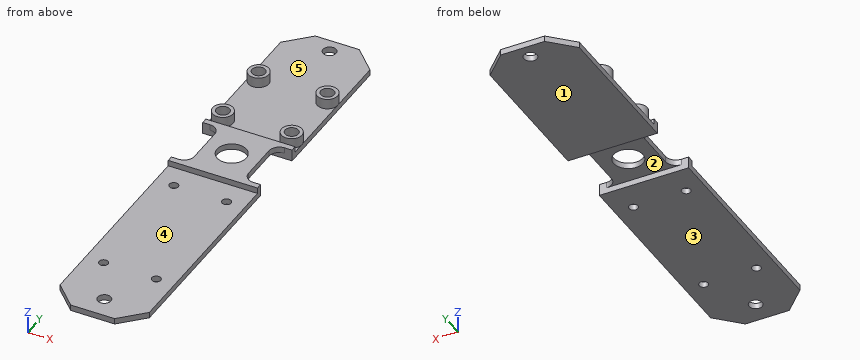
from build123d import *

# Parameters (mm, degrees)
SKETCH_1_W                   = 157.5
SKETCH_1_H                   = 30.5
EXTRUDE_1_DEPTH              = 2
HOLE_WIZARD_4_5_3_05_1_D     = 3.05
HOLE_WIZARD_4_5_3_05_1_DEPTH = 2.5
SKETCH_4_R                   = 3.5
EXTRUDE_2_DEPTH              = 3.5
SKETCH_5_R                   = 2.275
CUT_EXTRUDE_1_DEPTH          = 3.5
SKETCH_6_W                   = 30.5
SKETCH_6_H                   = 20.2
CUT_EXTRUDE_3_DEPTH          = 2.1
SKETCH_9_W                   = 30.5
SKETCH_9_H                   = 24.2
EXTRUDE_6_DEPTH              = 2
SKETCH_12_R                  = 5
CUT_EXTRUDE_4_DEPTH          = 6.5
HOLE_WIZARD_M4_1_D           = 4.5
SKETCH_13_W                  = 6
SKETCH_13_H                  = 20.2
CUT_EXTRUDE_5_DEPTH          = 4.5
FILLET_8_R                   = 3.5
CHAMFER_1_SIZE               = 7.75


with BuildPart() as part:
    # ｽｹｯﾁ1 → ﾎﾞｽ - 押し出し1 (new body)
    with BuildSketch(Plane(origin=(0, 0, 0), x_dir=(0, 1, 0), z_dir=(0, 0, 1))):
        with Locations((78.75, 15.25)):
            Rectangle(SKETCH_1_W, SKETCH_1_H)
    extrude(amount=EXTRUDE_1_DEPTH)

    # Ø4.5 (3.05) 直径の穴1
    with Locations(Plane.XY.offset(2)):
        with Locations((-24.25, 24), (-6.25, 69.2), (-24.25, 69.2), (-6.25, 24)):
            Hole(HOLE_WIZARD_4_5_3_05_1_D / 2, depth=HOLE_WIZARD_4_5_3_05_1_DEPTH)

    # ｽｹｯﾁ4 → ﾎﾞｽ - 押し出し2 (add)
    with BuildSketch(Plane.XY.offset(2)):
        with Locations((-27, 129)):
            Circle(SKETCH_4_R)
        with Locations((-3.5, 129)):
            Circle(SKETCH_4_R)
        with Locations((-3.5, 106)):
            Circle(SKETCH_4_R)
        with Locations((-27, 106)):
            Circle(SKETCH_4_R)
    extrude(amount=EXTRUDE_2_DEPTH)

    # ｽｹｯﾁ5 → ｶｯﾄ - 押し出し1 (cut)
    with BuildSketch(Plane.XY.offset(5.5)):
        with Locations((-27, 129)):
            Circle(SKETCH_5_R)
        with Locations((-3.5, 129)):
            Circle(SKETCH_5_R)
        with Locations((-3.5, 106)):
            Circle(SKETCH_5_R)
        with Locations((-27, 106)):
            Circle(SKETCH_5_R)
    extrude(amount=-CUT_EXTRUDE_1_DEPTH, mode=Mode.SUBTRACT)

    # ｽｹｯﾁ6 → ｶｯﾄ - 押し出し3 (cut)
    with BuildSketch(Plane(origin=(0, 0, 0), x_dir=(1, 0, 0), z_dir=(0, 0, -1))):
        with Locations((-15.25, -89.5)):
            Rectangle(SKETCH_6_W, SKETCH_6_H)
    extrude(amount=-CUT_EXTRUDE_3_DEPTH, mode=Mode.SUBTRACT)

    # ｽｹｯﾁ9 → ﾎﾞｽ - 押し出し6 (add)
    with BuildSketch(Plane.XY.offset(2)):
        with Locations((-15.25, 89.5)):
            Rectangle(SKETCH_9_W, SKETCH_9_H)
    extrude(amount=EXTRUDE_6_DEPTH)

    # ｽｹｯﾁ12 → ｶｯﾄ - 押し出し4 (cut, through all)
    with BuildSketch(Plane.XY.offset(5.5)):
        with Locations((-15.25, 89.5)):
            Circle(SKETCH_12_R)
    extrude(amount=-CUT_EXTRUDE_4_DEPTH, mode=Mode.SUBTRACT)

    # M4 すきま穴1 (through all)
    with Locations(Plane.XY.offset(2)):
        with Locations((-15.25, 152.5), (-15.25, 7.5)):
            Hole(HOLE_WIZARD_M4_1_D / 2)

    # ｽｹｯﾁ13 → ｶｯﾄ - 押し出し5 (cut, through all)
    with BuildSketch(Plane(origin=(0, 0, 2), x_dir=(1, 0, 0), z_dir=(0, 0, -1))):
        with Locations((-3, -89.5)):
            Rectangle(SKETCH_13_W, SKETCH_13_H)
        with Locations((-27.5, -89.5)):
            Rectangle(SKETCH_13_W, SKETCH_13_H)
    extrude(amount=-CUT_EXTRUDE_5_DEPTH, mode=Mode.SUBTRACT)

    # ﾌｨﾚｯﾄ8
    fillet_8_edges = [part.edges().sort_by_distance(p)[0] for p in [
        (-6, 99.6, 3),
        (-6, 79.4, 3),
        (-24.5, 79.4, 3),
        (-24.5, 99.6, 3),
    ]]
    fillet(fillet_8_edges, radius=FILLET_8_R)

    # 面取り1
    chamfer_1_edges = [part.edges().sort_by_distance(p)[0] for p in [
        (0, 157.5, 1),
        (-30.5, 157.5, 1),
        (-30.5, 0, 1),
        (0, 0, 1),
    ]]
    chamfer(chamfer_1_edges, length=CHAMFER_1_SIZE)


solid = part.part
The listing builds one solid part. Answer for the finished solid, in the listing's coordinates (mm). Face numbers are marked on the shaded views. A direction names the side the tool comes from. Give positions to 0.01 mm unless a question says otherwise; leave off trailing zeros. Write each loop counter-clockwise with the first axis right and the second up, starting at its lowest first coordinate (ties: lowest second). Pieces come first, ordered by that corner, then holes. Notation, with made-up numbers: (-39.5, -4) -> (-18.5, -4) arc R20 cw to (-18.5, 32) -> close; hole circle Ø3 at (66, 23.25). An arc over 180 degrees is marked (long way). One line per question, with ' | ' between items. Start each with the question number.
1. Section A-A (y = 89.5) is taken. Determine the outline of the cut face in (x, z), plus the area to 3 significant figures.
2. Section D-D (y = 142.5) is taken. Determine the outline of the cut face in (x, z), plus the area to 3 significant figures.
3. For a pull along Y with two mould halves and no side action, classify the marked faces 1 and 2 as pulls with the +Y half, pulls with the -Y half, needs draft (parallel to the pull), parting line crosses it, or undercut.
4. Find the intervals of material crossed by probe 1 along Y at (x, z) = (-15.25, 0.7); probe 2 along Y at (x, z) = (-5, 1.6); probe 3 along Y at (x, z) = (-22.5, 1.6), in increasing order.
5. For the marked faces 3, 4 and 5, determine the directions among +Z, -Z, +X, -X, +Y, -Y from which every point of the face is accessible in a straight line to the end or side of a thin tool.
6. Section B-B (z = 1.1) is taken. Determine the outline of the cut face in (x, y) (3 decimals).
7. Given pin 1 Ø10 at (x, y) = (-6.5, 84.5) entering from +Z; pin 2 Ø1.6 at (x, z) = (-22, 3) entering from -Y; pin 3 Ø0.6 at (y, z) = (89, 2.5) entering from +X, each flat-ended and moving along its own axis, determine where each tip first touches the part or whether it passes through.
8. Section C-C (y = 24) is taken. Determine the outline of the cut face in (x, z) (3 decimals), plus the area to 3 significant figures.
Response values:
1) outline: (-24.5, 2) -> (-20.25, 2) -> (-20.25, 4) -> (-24.5, 4) -> close; (-10.25, 2) -> (-6, 2) -> (-6, 4) -> (-10.25, 4) -> close | area: 17.0 mm2
2) outline: (-30.5, 0) -> (0, 0) -> (0, 2) -> (-30.5, 2) -> close | area: 61.0 mm2
3) face 1: needs draft | face 2: undercut
4) probe 1: 0 to 5.25, 9.75 to 79.4, 99.6 to 150.25, 154.75 to 157.5 | probe 2: 2.75 to 23.13, 24.87 to 68.33, 70.07 to 79.4, 99.6 to 154.75 | probe 3: 0 to 79.4, 99.6 to 157.5
5) face 3: -Z, +X, -X, +Y, -Y | face 4: +Z, +X, -X, -Y | face 5: +Z
6) outline: (-30.5, 7.75) -> (-22.75, 0) -> (-7.75, 0) -> (0, 7.75) -> (0, 79.4) -> (-30.5, 79.4) -> close; (-30.5, 99.6) -> (0, 99.6) -> (0, 149.75) -> (-7.75, 157.5) -> (-22.75, 157.5) -> (-30.5, 149.75) -> close; hole circle Ø3.05 at (-24.25, 24); hole circle Ø3.05 at (-24.25, 69.2); hole circle Ø4.5 at (-15.25, 7.5); hole circle Ø4.5 at (-15.25, 152.5); hole circle Ø3.05 at (-6.25, 24); hole circle Ø3.05 at (-6.25, 69.2)
7) pin 1: z = 4 | pin 2: y = 77.4 | pin 3: x = -6
8) outline: (-30.5, 0) -> (-25.775, 0) -> (-25.775, 2) -> (-30.5, 2) -> close; (-22.725, 0) -> (-7.775, 0) -> (-7.775, 2) -> (-22.725, 2) -> close; (-4.725, 0) -> (0, 0) -> (0, 2) -> (-4.725, 2) -> close | area: 48.8 mm2
